For this review, take the finished solid that the model builds, in its own axes (mm). Round coordinates to 2 decimals unless told otherwise and drop trailing zeros. Order: outer loops, then holes, each group sorted by start corner. A loop starts at its lowest first (then second) coordinate and runs counter-clockwise, first axis right, second up. Notation, with made-up numbers: (9.5, 73.25) -> (63.5, 73.25) arc R7 cw to (63.5, 85.25) -> close; hole circle Ø11 at (87, -19.75). An arc over 180 degrees is marked (long way). Use a Markdown table: item, result. Add a question column.
1) Draft analysis for pull direction X (two halves, no side actions). For faces 1 (the face through (-4.1, -15, -3.4)), 2 (the face through (7.677, -7.395, 6.634)), 3 (the face through (-7.589, -7.395, 6.634)), 4 (the face through (17.5, -7, 0)), state which applies: pulls with the +X half, pulls with the -X half, needs draft (parallel to the pull), parting line crosses it, or undercut.
2) Clearance check with a flat-ended pin moving along its axis: P1, Ø1.2, axis at x = 7.633, z = 7.633, coming from the +Y side. State where the tip first meets the part, or that it passes through.
3) Consider section B-B (y = -7.5). State the section outline as (x, z) points, plus the area to 3 significant figures.
4) Consider section D-D (y = -13.75). State the section outline as (x, z) points, plus the area to 3 significant figures.
5) Consider section A-A (z = 0). State the section outline as (x, y) points.
6) Consider section C-C (x = 0). State the section outline as (y, z) points.
7) Wall thickness on line 1 along Z through (x, y) = (-7.5, -13.75); line 2 along Z through (x, y) = (-9.5, -7.5); line 3 along X through (y, z) = (-10, 7): over which ranges is each line inside the solid? List them lowest first. Write a range as [from, to].
```python
from build123d import *

# Parameters (mm, degrees)
SKETCH1_W             = 35
SKETCH1_H             = 28.575
BOSS_EXTRUDE1_DEPTH   = 15
SKETCH2_R             = 5.08
CUT_EXTRUDE2_DEPTH    = 30
SKETCH4_R             = 1
CUT_EXTRUDE3_DEPTH    = 15
M4X0_7_TAPPED_HOLE1_D = 3.3


with BuildPart() as part:
    # Sketch1 → Boss-Extrude1 (new body)
    with BuildSketch(Plane(origin=(0, 0, 0), x_dir=(1, 0, 0), z_dir=(0, 1, 0))):
        Rectangle(SKETCH1_W, SKETCH1_H)
    extrude(amount=-BOSS_EXTRUDE1_DEPTH)

    # Sketch2 → Cut-Extrude2 (cut)
    with BuildSketch(Plane(origin=(0, 0, 0), x_dir=(1, 0, 0), z_dir=(0, 1, 0))):
        with Locations(Location((0, 0, 0), (0, 0, 270))):
            Circle(SKETCH2_R)
    extrude(amount=-CUT_EXTRUDE2_DEPTH, mode=Mode.SUBTRACT)

    # Sketch4 → Cut-Extrude3 (cut)
    with BuildSketch(Plane(origin=(0, 0, 0), x_dir=(1, 0, 0), z_dir=(0, 1, 0))):
        with Locations(Location((7.633, 7.633, 0), (0, 0, 270))):
            Circle(SKETCH4_R)
        with Locations(Location((-7.633, 7.633, 0), (0, 0, 270))):
            Circle(SKETCH4_R)
        with Locations(Location((-7.633, -7.633, 0), (0, 0, 270))):
            Circle(SKETCH4_R)
        with Locations(Location((7.633, -7.633, 0), (0, 0, 270))):
            Circle(SKETCH4_R)
    extrude(amount=-CUT_EXTRUDE3_DEPTH, mode=Mode.SUBTRACT)

    # M4x0.7 Tapped Hole1 (through all)
    with Locations(Plane(origin=(-17.5, 0, 0), x_dir=(0, -1, 0), z_dir=(-1, 0, 0))):
        with Locations((7.5, -9.2875), (7.5, 9.2875)):
            Hole(M4X0_7_TAPPED_HOLE1_D / 2)


solid = part.part
```
Results list:
| question | item | result |
|---|---|---|
| 1 | face 1 | needs draft |
| 1 | face 2 | undercut |
| 1 | face 3 | undercut |
| 1 | face 4 | pulls with the +X half |
| 2 | P1 | through |
| 3 | outline | (-17.5, -14.29) -> (17.5, -14.29) -> (17.5, -10.94) -> (-17.5, -10.94) -> close; (-17.5, -7.64) -> (-8.63, -7.64) arc R1 cw (long way) to (-6.63, -7.64) -> (6.63, -7.64) arc R1 cw (long way) to (8.63, -7.64) -> (17.5, -7.64) -> (17.5, 7.64) -> (8.63, 7.64) arc R1 cw (long way) to (6.63, 7.64) -> (-6.63, 7.64) arc R1 cw (long way) to (-8.63, 7.64) -> (-17.5, 7.64) -> close; (-17.5, 10.94) -> (17.5, 10.94) -> (17.5, 14.29) -> (-17.5, 14.29) -> close; hole circle Ø10.16 at (0, 0) |
| 3 | area | 682 mm2 |
| 4 | outline | (-17.5, -14.29) -> (17.5, -14.29) -> (17.5, 14.29) -> (-17.5, 14.29) -> close; hole circle Ø2 at (-7.63, -7.63); hole circle Ø2 at (-7.63, 7.63); hole circle Ø10.16 at (0, 0); hole circle Ø2 at (7.63, -7.63); hole circle Ø2 at (7.63, 7.63) |
| 4 | area | 906 mm2 |
| 5 | outline | (-17.5, -15) -> (-5.08, -15) -> (-5.08, 0) -> (-17.5, 0) -> close; (5.08, -15) -> (17.5, -15) -> (17.5, 0) -> (5.08, 0) -> close |
| 6 | outline | (-15, -14.29) -> (0, -14.29) -> (0, -5.08) -> (-15, -5.08) -> close; (-15, 5.08) -> (0, 5.08) -> (0, 14.29) -> (-15, 14.29) -> close; hole circle Ø3.3 at (-7.5, -9.29); hole circle Ø3.3 at (-7.5, 9.29) |
| 7 | line 1 | [-14.29, -8.62], [-6.64, 6.64], [8.62, 14.29] |
| 7 | line 2 | [-14.29, -10.94], [-7.64, 7.64], [10.94, 14.29] |
| 7 | line 3 | [-17.5, -8.41], [-6.86, 6.86], [8.41, 17.5] |
